Autodesk Inventor part; units mm, degrees
ref_plane "Work Plane1" through (30.1625, 0, 0) normal (0, 0, -1) x (1, 0, 0)
ref_plane "YZ Plane" through (0, 0, 0) normal (1, 0, 0) x (0, 1, 0)
ref_plane "XZ Plane" through (0, 0, 0) normal (0, 1, 0) x (-1, 0, 0)
sketch "Sketch1" plane through (0, 0, 0) normal (0, 0, 1) x (1, 0, 0)
  line L0 (-1.3, 0) -> (6, 0)
  line L1 (6, 0) -> (6, 1)
  line L2 (6, 1) -> (0.4, 1)
  line L3 (0.4, 1) -> (0.1545, 1)
  line L4 (0.1545, 1) -> (0, 1)
  line L5 (0, 1) -> (0, 2)
  line L6 (-2.76, 0) -> (7.46, 0)
  line L7 (0, -0.4) -> (0, 2.4)
  line L8 (-1.3, 0) -> (-1.3, 2)
  line L9 (0, 2) -> (-1.3, 2)
  line L10 (0.4, 1) -> (0, 1) construction
  dimension "d0" = 6
  dimension "d1" = 5.6
  dimension "d2" = 0.2455
  dimension "d3" = 1.3
  dimension "d4" = 2
  dimension "d5" = 2
  dimension "d9" = 4
  dimension "d10" = 0
revolve "Body" add sketch "Sketch1" angle 360 about axis through (-1.3, 0, 0) along (1, 0, 0)
sketch "Sketch2" plane through (-1.3, 0, 0) normal (-1, 0, 0) x (0, 0, 1)
  circle A0 centre (0, 0) radius 2
  line L0 (0, 0) -> (0, 2)
  line L1 (-2, 0.35) -> (2, 0.35)
  line L2 (2, 0.35) -> (2, -0.35)
  line L3 (2, -0.35) -> (-2, -0.35)
  line L4 (-2, -0.35) -> (-2, 0.35)
  line L5 (-2, 0) -> (2, 0) construction
  line L6 (0, 0.35) -> (0, -0.35) construction
  dimension "d11" = 0.7
  dimension "d12" = 4
fillet "Fillet1" radius 0.8 1 edges at (-1.3, -2, 0)
extrude "Slot" cut sketch "Sketch2" against normal blind 0.5 contours A0 L3 L1 | L2 L3 A0 | A0 L1 L2 | L3 L4 A0 | A0 L4 L1
thread "Thread"
chamfer "Chamfer1" distance 0.335 distance2 0.2455 1 edges at (6, -1, 0) measured on face at (6, 0.2495, 0.221)
ref_plane "Work Plane1" through (30.1625, 0, 0) normal (0, 0, -1) x (1, 0, 0)
fillet "Fillet2" radius 0.1 1 edges at (0, -1, 0)
equation "\"d11\" = SBR"
equation "\"d12\" = KOD"
equation "\"d14\" = RR"
equation "\"d19\" = STI"
equation "\"d15\" = GEL"
equation "\"d17\" = -0.5 * SPD + 0.5 * GD"
equation "\"d40\" = R"
equation "\"d0\" = NLG"
equation "\"d1\" = GEL"
equation "\"d3\" = KOH"
equation "\"d4\" = GD"
equation "\"d5\" = BDM"
equation "\"d9\" = KOD"
equation "\"GD\" = NND"
equation "\"NLG\" = 6"
equation "\"GEL\" = 5.6"
equation "\"KOD\" = 4"
equation "\"KOH\" = 1.3"
equation "\"GAL\" = 0.61345 * PTC"
equation "\"SPD\" = 1.33"
equation "\"BDM\" = NND"
equation "\"GUL\" = 0.61345 * PTC"
equation "\"RR\" = 0.8"
equation "\"SBR\" = 0.7"
equation "\"STI\" = 0.5"
equation "\"KEWI\" = 0"
equation "\"R\" = 0.1"
equation "\"PTC\" = 0.4"
equation "\"THREADDIA\" = 2"
equation "\"TOA\" = 30deg"
equation "\"NND\" = 2"
equation "\"GD1\" = THREADDIA - 1.2269 * PTC"
properties part number "ANSI B18.6.7M - M2x0.4 x 6" material "Steel, Mild"
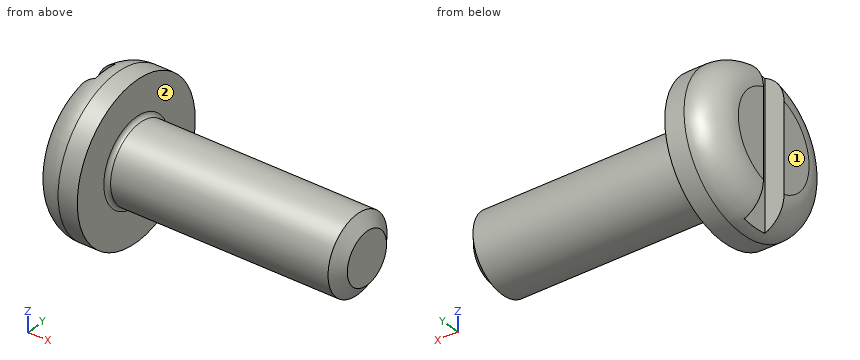
For this review, take the finished solid that the model builds, in its own axes (mm). Face numbers are marked on the shaded views. A direction names the side the tool comes from. Round coordinates to 2 decimals unless told otherwise and drop trailing zeros. Write each loop counter-clockwise with the first axis right and the second up, starting at its lowest first coordinate (ties: lowest second). Pieces come first, ordered by that corner, then holes. Notation, with made-up numbers: (80.25, 36) -> (134.25, 36) arc R33 ccw to (134.25, 70) -> close; hole circle Ø9 at (20, 39). An arc over 180 degrees is marked (long way). One line per question, with ' | ' between items. Start each with the question number.
1) Wall thickness on line 1 along X through (y, z) = (-0.3, -1.75); line 2 along X through (y, z) = (-0.2, -0.15); line 3 along Z through (x, y) = (5.25, -0.35): over which ranges is each line inside the solid? List them lowest first.
2) Machinability: for the marked faces 1 and 2, which of the approach directions +Z, -Z, +X, -X, +Y, -Y give a long, thin tool a straight path to every point of the face, cutting with its end or side? Answer none if there is none.
3) Add section C-C (x = 5.5). Write out the cut boundary in (y, z), and give its area (3 significant figures).
4) For pin 1 Ø2 at (x, y) = (1.5, -1.5) entering from -Z; pin 2 Ø2 at (x, z) = (3, -0.5) entering from -Y; pin 3 Ø2 at (y, z) = (-1, -0.5) entering from +X, all flat-tipped, find the tip position at first contact; note any pin that passes through.
Reported:
1) line 1: x = -0.8 to 0 | line 2: x = -0.8 to 6 | line 3: z = -0.94 to 0.94
2) face 1: +Z, -Z, -X, +Y, -Y | face 2: +X
3) outline: circle Ø2 at (0, 0) | area: 3.14 mm²
4) pin 1: stops at z = -0.87 | pin 2: stops at y = -1 | pin 3: stops at x = 6
